For this review, take the finished solid that the model builds, in its own axes (mm). Face numbers are marked on the shaded views. Round coordinates to 2 decimals unless told otherwise and drop trailing zeros. Write each loop counter-clockwise with the first axis right and the second up, starting at its lowest first coordinate (ties: lowest second). Pieces come first, ordered by that corner, then holes. Notation, with made-up numbers: (-16, -37) -> (5, -37) arc R11 cw to (5, -31) -> close; hole circle Ø9 at (77.25, 50). An arc over 180 degrees is marked (long way). Answer as CSV lines item,"result". Start each with the question number.
Item 1: Wall thickness on probe 1 along X at (y, z) = (6, 0) (3 decimals); probe 2 along Y at (x, z) = (38, -2); probe 3 along X at (y, z) = (5.75, 12.5): over which ranges is each line inside the solid? List them lowest first. Write a range as from..to.
Item 2: Take a section at C-C on y = 8.5. Give the boundary of the cut face in (x, z) (3 decimals), then the cut area to 3 significant figures.
Item 3: Take a section at B-B on x = 0. Give the boundary of the cut face in (y, z) (3 decimals).
Item 4: Mouldability with a two-part tool opening along Z and no side actions: class the marked faces 1, 2 and 3 as +Z half, -Z half, draft (parallel to the pull), parting line (faces both ways), or undercut.
Item 5: Take a section at A-A on z = 0. Give the boundary of the cut face in (x, y) (3 decimals), then the cut area to 3 significant figures.
Item 6: For pin 1 Ø1 at (y, z) = (5.5, -20) entering from -X; pin 2 Ø3 at (x, y) = (-6.5, 17.5) entering from -Z; pin 3 Ø12 at (x, z) = (6, 9) entering from -Y; pin 4 Ø10 at (x, z) = (4.5, -1) entering from -Y, all flat-tipped, find the tip position at first contact; note any pin that passes through.
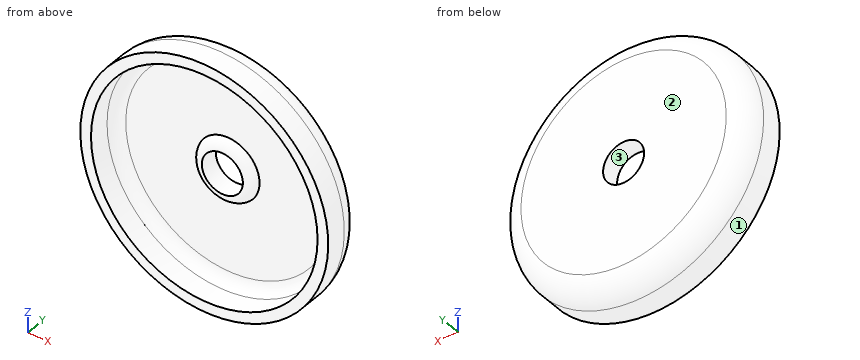
```python
from build123d import *

# Parameters (mm, degrees)
SKETCH1_R           = 59.055
BOSS_EXTRUDE1_DEPTH = 20.32
SKETCH2_R           = 9.779
CUT_EXTRUDE1_DEPTH  = 86.952826888
FILLET1_R           = 10.16
SHELL2_T            = -5.08
CUT_EXTRUDE3_START  = -11.43
SKETCH4_R           = 14.859
SKETCH4_R_2         = 9.779
CUT_EXTRUDE3_DEPTH  = 11.43
FILLET3_R           = 5.08


with BuildPart() as part:
    # Sketch1 → Boss-Extrude1 (new body)
    with BuildSketch(Plane(origin=(0, 0, 0), x_dir=(1, 0, 0), z_dir=(0, 1, 0))):
        with Locations(Location((0, 0, 0), (0, 0, 270))):
            Circle(SKETCH1_R)
    extrude(amount=BOSS_EXTRUDE1_DEPTH)

    # Sketch2 → Cut-Extrude1 (cut, through all)
    with BuildSketch(Plane(origin=(0, 20.32, 0), x_dir=(1, 0, 0), z_dir=(0, 1, 0))):
        with Locations(Location((0, 0, 0), (0, 0, 270))):
            Circle(SKETCH2_R)
    extrude(amount=-CUT_EXTRUDE1_DEPTH, mode=Mode.SUBTRACT)

    # Fillet1
    fillet1_edges = [part.edges().sort_by_distance(p)[0] for p in [
        (0, 20.32, -59.055),
    ]]
    fillet(fillet1_edges, radius=FILLET1_R)

    # Shell2
    shell2_openings = [part.faces().sort_by_distance(p)[0] for p in [
        (0, 0, -57.384672361),
    ]]
    offset(amount=SHELL2_T, openings=shell2_openings, kind=Kind.INTERSECTION)

    # Sketch4 → Cut-Extrude3 (cut)
    with BuildSketch(Plane.XZ.offset(CUT_EXTRUDE3_START)):
        with Locations(Location((0, 0, 0), (0, 0, 90))):
            Circle(SKETCH4_R)
        with Locations(Location((0, 0, 0), (0, 0, 90))):
            Circle(SKETCH4_R_2, mode=Mode.SUBTRACT)
    extrude(amount=CUT_EXTRUDE3_DEPTH, mode=Mode.SUBTRACT)

    # Fillet3
    # the kernel refuses this fillet: 5.08 mm, written as the material it takes off along each edge
    with BuildSketch(Plane(origin=(0, 11.43, 0), x_dir=(0, 0, 1), z_dir=(1, 0, 0))) as fillet3_piece_1:
        with BuildLine():
            CenterArc((9.94031115, -5.08), FILLET3_R, 14.477512186, 75.522487814)
            Line((14.859, -3.81), (14.957373777, -3.7846))
            ThreePointArc((14.957373777, -3.7846), (14.9606, -1.905), (14.9606, 0))
            Line((14.9606, 0), (14.859, 0.1016))
            Line((14.859, 0.1016), (9.94031115, 0.1016))
            Line((9.94031115, 0.1016), (9.94031115, 0))
        make_face()
    revolve(axis=Axis((0, 11.43, 0), (0, -1, 0)), mode=Mode.SUBTRACT)


solid = part.part
```
Output values:
1,probe 1,"x = -59.055..-53.975, 53.975..59.055"
1,probe 2,"y = 15.24..20.32"
1,probe 3,"x = -57.72..-52.51, 52.51..57.72"
2,outline,"circle Ø118.11 at (0, 0); hole circle Ø107.95 at (0, 0)"
2,area,"1,800 mm^2"
3,outline,"(0, -59.055) -> (10.16, -59.055) arc R10.16 ccw to (20.32, -48.895) -> (20.32, -9.779) -> (11.43, -9.779) -> (11.43, -9.94) arc R5.08 ccw to (15.24, -14.859) -> (15.24, -48.895) arc R5.08 cw to (10.16, -53.975) -> (0, -53.975) -> close; (0, 53.975) -> (10.16, 53.975) arc R5.08 cw to (15.24, 48.895) -> (15.24, 14.859) arc R5.08 ccw to (11.43, 9.94) -> (11.43, 9.779) -> (20.32, 9.779) -> (20.32, 48.895) arc R10.16 ccw to (10.16, 59.055) -> (0, 59.055) -> close"
4,face 1,"parting line"
4,face 2,"draft"
4,face 3,"undercut"
5,outline,"(-59.055, 0) -> (-53.975, 0) -> (-53.975, 10.16) arc R5.08 cw to (-48.895, 15.24) -> (-14.859, 15.24) arc R5.08 ccw to (-9.94, 11.43) -> (-9.779, 11.43) -> (-9.779, 20.32) -> (-48.895, 20.32) arc R10.16 ccw to (-59.055, 10.16) -> close; (9.779, 11.43) -> (9.94, 11.43) arc R5.08 ccw to (14.859, 15.24) -> (48.895, 15.24) arc R5.08 cw to (53.975, 10.16) -> (53.975, 0) -> (59.055, 0) -> (59.055, 10.16) arc R10.16 ccw to (48.895, 20.32) -> (9.779, 20.32) -> close"
5,area,"651 mm^2"
6,pin 1,"stops at x = -55.74"
6,pin 2,"stops at z = -56.85"
6,pin 3,"stops at y = 11.43"
6,pin 4,"passes through"
